from build123d import *

# Parameters (mm, degrees)
SKETCH1_W           = 70
SKETCH1_H           = 70
BOSS_EXTRUDE1_DEPTH = 10
SKETCH2_R           = 1.65
CUT_EXTRUDE1_DEPTH  = 10
SKETCH3_R           = 4
CUT_EXTRUDE2_DEPTH  = 5


with BuildPart() as part:
    # Sketch1 → Boss-Extrude1 (new body)
    with BuildSketch(Plane(origin=(0, 0, 0), x_dir=(1, 0, 0), z_dir=(0, 1, 0))):
        Rectangle(SKETCH1_W, SKETCH1_H)
    extrude(amount=BOSS_EXTRUDE1_DEPTH)

    # Sketch2 → Cut-Extrude1 (cut)
    with BuildSketch(Plane(origin=(0, 10, 0), x_dir=(1, 0, 0), z_dir=(0, 1, 0))):
        with Locations(Location((-13, 13, 0), (0, 0, 270))):
            Circle(SKETCH2_R)
        with Locations(Location((13, 13, 0), (0, 0, 90))):
            Circle(SKETCH2_R)
        with Locations(Location((13, -13, 0), (0, 0, 270))):
            Circle(SKETCH2_R)
        with Locations(Location((-13, -13, 0), (0, 0, 90))):
            Circle(SKETCH2_R)
    extrude(amount=-CUT_EXTRUDE1_DEPTH, mode=Mode.SUBTRACT)

    # Sketch3 → Cut-Extrude2 (cut)
    with BuildSketch(Plane(origin=(0, 10, 0), x_dir=(1, 0, 0), z_dir=(0, 1, 0))):
        with Locations(Location((0, 0, 0), (0, 0, 270))):
            Circle(SKETCH3_R)
    extrude(amount=-CUT_EXTRUDE2_DEPTH, mode=Mode.SUBTRACT)


solid = part.part
Read the model definition and answer for the solid it produces. Units are mm, in the model's axes. A direction names the side the tool comes from. Coordinates: 2 decimals unless noted, no trailing zeros. Loops run counter-clockwise (first coordinate to the right, second up) from the corner with the lowest first, then second, coordinate; pieces in that order, holes last.
Q1. The part is cut by section B-B on y = 7.5. Write down the section's boundary in (x, z).
Q2. The part is cut by section A-A on x = -13. Write down the section's boundary in (y, z), and give its area (3 significant figures).
Q3. The part is cut by section D-D on x = 0. Write down the section's boundary in (y, z), and give its area (3 significant figures).
Q4. The part is cut by section C-C on z = 0. Write down the section's boundary in (x, y), and give its area (3 significant figures).
Q5. This flat-tipped pin is pushed along its axis until it touches: pin 1 Ø10.5 at (x, z) = (0, 0) entering from +Y. Where does it stop, or does it pass through?
Q6. The mould has two halves that part along X. Classify faces 3 (the face through (7, 10, 0)), 4 (the face through (-35, 5, 0)), 5 (the face through (-3.905, 7.535, -0.867)): +X half, -X half, draft (parallel to the pull), parting line (faces both ways), or undercut.
Q7. Which of the six approach directions +Z, -Z, +X, -X, +Y, -Y give full straight-line access (tool end or side, diameter ignored) to faces 1 (the face through (0, 5, 0)), 2 (the face through (0, 5, 35))?
Q8. Consider probe 1 along X at (y, z) = (8, 13); probe 2 along X at (y, z) = (4, 14). Determine where each line is inside the solid, lowest interval first.
Results below:
1. outline: (-35, -35) - (35, -35) - (35, 35) - (-35, 35) - close; hole circle Ø3.3 at (-13, -13); hole circle Ø3.3 at (-13, 13); hole circle Ø8 at (0, 0); hole circle Ø3.3 at (13, -13); hole circle Ø3.3 at (13, 13)
2. outline: (0, -35) - (10, -35) - (10, -14.65) - (0, -14.65) - close; (0, -11.35) - (10, -11.35) - (10, 11.35) - (0, 11.35) - close; (0, 14.65) - (10, 14.65) - (10, 35) - (0, 35) - close
2. area: 634 mm2
3. outline: (0, -35) - (10, -35) - (10, -4) - (5, -4) - (5, 4) - (10, 4) - (10, 35) - (0, 35) - close
3. area: 660 mm2
4. outline: (-35, 0) - (35, 0) - (35, 10) - (4, 10) - (4, 5) - (-4, 5) - (-4, 10) - (-35, 10) - close
4. area: 660 mm2
5. pin 1: stops at y = 10
6. face 3: draft
6. face 4: -X half
6. face 5: undercut
7. face 1: +Y
7. face 2: +Z, +X, -X, +Y, -Y
8. probe 1: x = -35 to -14.65, -11.35 to 11.35, 14.65 to 35
8. probe 2: x = -35 to -14.31, -11.69 to 11.69, 14.31 to 35
